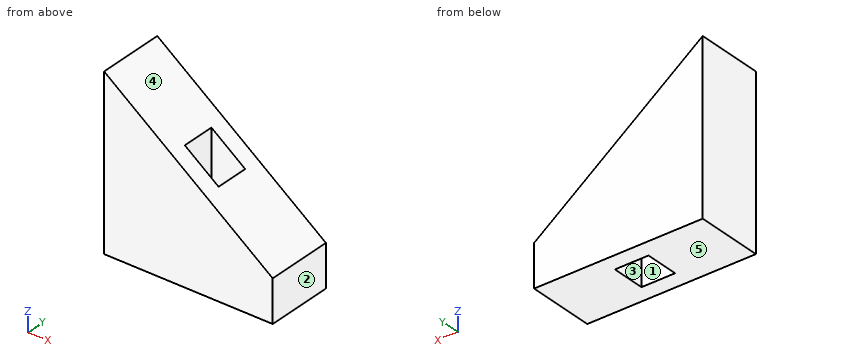
from build123d import *

# Parameters (mm, degrees)
F1_DEPTH = 40
F2_W     = 20
F2_H     = 20
F3_DEPTH = 100.001


with BuildPart() as f1:
    # F0 (on Front) → F1 (new body)
    with BuildSketch(Plane.XZ):
        Polygon((0, 100), (0, 0), (100, 0), (100, 25), align=None)
    extrude(amount=F1_DEPTH)

    # F2 (on face) → F3 (cut, through all)
    with BuildSketch(Plane(origin=(0, 0, 0), x_dir=(1, 0, 0), z_dir=(0, 0, -1))):
        with Locations((50, 20)):
            Rectangle(F2_W, F2_H)
    extrude(amount=-F3_DEPTH, mode=Mode.SUBTRACT)


solid = f1.part
Geometry: final body of the model. Coordinates: model frame, mm. Face numbers are marked on the shaded views. A direction names the side the tool comes from. Give positions to 0.01 mm unless a question says otherwise; leave off trailing zeros. Order: outer loops, then holes, each group sorted by start corner. A loop starts at its lowest first (then second) coordinate and runs counter-clockwise, first axis right, second up. Notation, with made-up numbers: (-25.75, 15) -> (16.25, 15) arc R10 ccw to (16.25, 19) -> close; hole circle Ø4 at (-27.5, -6.75). An arc over 180 degrees is marked (long way). Write each question's results on one line, items separated by ' | '.
1) Draft query along X for the marked faces 3, 4 and 5. Return one class per face: released by +X, released by -X, zero draft, split by the parting line, or undercut.
Geometry says:
face 3: undercut | face 4: released by +X | face 5: zero draft
2) Cut plane D-D (z = 27). Output: boundary loops of the cut face in (x, y), and give its area (3 significant figures).
Geometry says:
outline: (0, -40) -> (97.33, -40) -> (97.33, 0) -> (0, 0) -> close; hole (40, -30) -> (60, -30) -> (60, -10) -> (40, -10) -> close | area: 3,490 mm²
3) First-contact query: pin 1 Ø22 at (y, z) = (-15.5, 29.5) entering from -X; pin 2 Ø4 at (y, z) = (-15, 69.5) entering from +X; pin 3 Ø5 at (y, z) = (-18.5, 54.5) entering from +X; pin 4 Ø16 at (y, z) = (-24.5, 42) entering from +X. Flat tips, straight axial feed; report the tip coordinate or a pass-through.
Geometry says:
pin 1: stops at x = 0 | pin 2: stops at x = 40 | pin 3: stops at x = 64 | pin 4: stops at x = 88
4) Cut plane C-C (z = 58). Output: boundary loops of the cut face in (x, y), and give its area (3 significant figures).
Geometry says:
outline: (0, -40) -> (56, -40) -> (56, -30) -> (40, -30) -> (40, -10) -> (56, -10) -> (56, 0) -> (0, 0) -> close | area: 1,920 mm²
5) Cut plane A-A (x = 50). Output: boundary loops of the cut face in (y, z).
Geometry says:
outline: (-40, 0) -> (-30, 0) -> (-30, 62.5) -> (-40, 62.5) -> close; (-10, 0) -> (0, 0) -> (0, 62.5) -> (-10, 62.5) -> close
6) Cut plane B-B (y = -11.5). Output: boundary loops of the cut face in (x, z), and give its area (3 significant figures).
Geometry says:
outline: (0, 0) -> (40, 0) -> (40, 70) -> (0, 100) -> close; (60, 0) -> (100, 0) -> (100, 25) -> (60, 55) -> close | area: 5,000 mm²
7) Set-up query: the marked faces 1 and 2. Return all of +Z, -Z, +X, -X, +Y, -Y with unobstructed straight access to the full face (end or side cutting, diameter ignored); none if empty.
Geometry says:
face 1: +Z, -Z | face 2: +Z, -Z, +X, +Y, -Y
8) Line query: line 1 along X through (y, z) = (-24, 17.5); line 2 along X through (y, z) = (-21.5, 49.5); line 3 along X through (y, z) = (-5, 86.5). Output: solid intervals per line, ascending.
Geometry says:
line 1: x = 0 to 40, 60 to 100 | line 2: x = 0 to 40, 60 to 67.33 | line 3: x = 0 to 18
